Model file for the job. Use its own axes, mm. Give positions to 0.01 mm unless a question says otherwise; leave off trailing zeros. Loops run counter-clockwise (first coordinate to the right, second up) from the corner with the lowest first, then second, coordinate; pieces in that order, holes last. Notation, with made-up numbers: M 37,-36.75 L 85,-36.75 A17 cw 85,-27.75 Z; hole C 28.5,-26 d5. An arc over 180 degrees is marked long. Use CSV: the item, a comma, the result in double quotes. Start each with the question number.
(1) Wall check: line 1 along X through (y, z) = (2.3, 12.7); line 2 along Z through (x, y) = (63.5, 0.7); line 3 along Z through (x, y) = (44, 1.85). Give the ranges that are in metal, low to high. Write a range as from..to.
(2) Slice it at B-B on x = 63.5. List the corners of the cut face in (y, z) (3 decimals), and give its area (3 significant figures).
(3) Slice it at A-A on z = 139.7. List the corners of the cut face in (x, y) (3 decimals).
(4) Two-plate mould, pull along X, no slides. Class faces 1 (the face through (25, 0, 98)), 2 (the face through (14.42, 1.61, 87.03)): pulls with the +X half, pulls with the -X half, needs draft (parallel to the pull), parting line crosses it, or undercut.
(5) Slice it at C-C on z = 114.3. List the corners of the cut face in (x, y) (3 decimals), and give its area (3 significant figures).
(6) Flat gauge pins, fed straight in: P1, Ø4.5, axis at x = 12.7, z = 63.5, coming from the +Y side (3 decimals); P2, Ø1, axis at y = 1, z = 62.5, coming from the +X side; P3, Ø1, axis at x = 87.5, y = 2, coming from the -Z side. Where does each tip first touch, or does it go through?
(7) Slice it at D-D on x = 12.7. List the corners of the cut face in (y, z) (3 decimals).
```python
from build123d import *

# Parameters (mm, degrees)
BOSS_EXTRUDE1_DEPTH = 3.175
SKETCH2_R           = 2.54
CUT_EXTRUDE1_DEPTH  = 3.175
LPATTERN1_COUNT     = 6
LPATTERN1_PITCH     = 25.4
SKETCH3_R           = 2.54
CUT_EXTRUDE2_DEPTH  = 3.175
LPATTERN2_COUNT     = 5
LPATTERN2_PITCH     = 25.4


with BuildPart() as part:
    # Sketch1 → Boss-Extrude1 (new body)
    with BuildSketch(Plane(origin=(0, 0, 0), x_dir=(1, 0, 0), z_dir=(0, 1, 0))):
        with BuildLine():
            Line((0, -2.54), (0, -149.86))
            ThreePointArc((0, -149.86), (0.743948776, -151.656051224), (2.54, -152.4))
            Line((2.54, -152.4), (149.86, -152.4))
            ThreePointArc((149.86, -152.4), (151.656051224, -151.656051224), (152.4, -149.86))
            Line((152.4, -149.86), (152.4, -129.54))
            ThreePointArc((152.4, -129.54), (151.656051224, -127.743948776), (149.86, -127))
            Line((149.86, -127), (27.94, -127))
            ThreePointArc((27.94, -127), (26.143948776, -126.256051224), (25.4, -124.46))
            Line((25.4, -124.46), (25.4, -2.54))
            ThreePointArc((25.4, -2.54), (24.656051224, -0.743948776), (22.86, 0))
            Line((22.86, 0), (2.54, 0))
            ThreePointArc((2.54, 0), (0.743948776, -0.743948776), (0, -2.54))
        make_face()
    extrude(amount=BOSS_EXTRUDE1_DEPTH)

    # Sketch2 → Cut-Extrude1 (cut)
    with BuildSketch(Plane(origin=(0, 3.175, 0), x_dir=(1, 0, 0), z_dir=(0, 1, 0))):
        with Locations(Location((12.7, -12.7, 0), (0, 0, 270))):
            Circle(SKETCH2_R)
    cut_extrude1 = extrude(amount=-CUT_EXTRUDE1_DEPTH, mode=Mode.SUBTRACT)

    # LPattern1: Cut-Extrude1 ×6
    with Locations(*[(0, 0, i * LPATTERN1_PITCH) for i in range(1, LPATTERN1_COUNT)]):
        add(cut_extrude1, mode=Mode.SUBTRACT)

    # Sketch3 → Cut-Extrude2 (cut)
    with BuildSketch(Plane(origin=(0, 3.175, 0), x_dir=(1, 0, 0), z_dir=(0, 1, 0))):
        with Locations(Location((139.7, -139.7, 0), (0, 0, 270))):
            Circle(SKETCH3_R)
    cut_extrude2 = extrude(amount=-CUT_EXTRUDE2_DEPTH, mode=Mode.SUBTRACT)

    # LPattern2: Cut-Extrude2 ×5
    with Locations(*[(-i * LPATTERN2_PITCH, 0, 0) for i in range(1, LPATTERN2_COUNT)]):
        add(cut_extrude2, mode=Mode.SUBTRACT)


solid = part.part
```
Reply:
1,line 1,"x = 0..10.16, 15.24..25.4"
1,line 2,"z = 127..137.16, 142.24..152.4"
1,line 3,"z = 127..152.4"
2,outline,"M 0,127 L 3.175,127 L 3.175,137.16 L 0,137.16 Z; M 0,142.24 L 3.175,142.24 L 3.175,152.4 L 0,152.4 Z"
2,area,"64.5 mm^2"
3,outline,"M 0,0 L 10.16,0 L 10.16,3.175 L 0,3.175 Z; M 15.24,0 L 35.56,0 L 35.56,3.175 L 15.24,3.175 Z; M 40.64,0 L 60.96,0 L 60.96,3.175 L 40.64,3.175 Z; M 66.04,0 L 86.36,0 L 86.36,3.175 L 66.04,3.175 Z; M 91.44,0 L 111.76,0 L 111.76,3.175 L 91.44,3.175 Z; M 116.84,0 L 137.16,0 L 137.16,3.175 L 116.84,3.175 Z; M 142.24,0 L 152.4,0 L 152.4,3.175 L 142.24,3.175 Z"
4,face 1,"needs draft"
4,face 2,"undercut"
5,outline,"M 0,0 L 10.16,0 L 10.16,3.175 L 0,3.175 Z; M 15.24,0 L 25.4,0 L 25.4,3.175 L 15.24,3.175 Z"
5,area,"64.5 mm^2"
6,P1,"passes through"
6,P2,"stops at x = 25.4"
6,P3,"stops at z = 127"
7,outline,"M 0,0 L 3.175,0 L 3.175,10.16 L 0,10.16 Z; M 0,15.24 L 3.175,15.24 L 3.175,35.56 L 0,35.56 Z; M 0,40.64 L 3.175,40.64 L 3.175,60.96 L 0,60.96 Z; M 0,66.04 L 3.175,66.04 L 3.175,86.36 L 0,86.36 Z; M 0,91.44 L 3.175,91.44 L 3.175,111.76 L 0,111.76 Z; M 0,116.84 L 3.175,116.84 L 3.175,137.16 L 0,137.16 Z; M 0,142.24 L 3.175,142.24 L 3.175,152.4 L 0,152.4 Z"
